```python
from build123d import *

# Parameters (mm, degrees)
SKETCH5_R           = 11
BOSS_EXTRUDE3_DEPTH = 3.84
SKETCH6_R           = 1.5
CUT_EXTRUDE16_DEPTH = 3.84
SKETCH6_8_R         = 2.9
SKETCH6_8_R_2       = 1.5
CUT_EXTRUDE17_DEPTH = 1
SKETCH7_R           = 0.75
CUT_EXTRUDE18_DEPTH = 2
SKETCH8_R           = 1.05
CUT_EXTRUDE20_DEPTH = 3
SKETCH8_4_R         = 1.25
SKETCH8_4_R_2       = 1.05
CUT_EXTRUDE21_DEPTH = 0.5
SKETCH15_W          = 0.299586516
SKETCH15_H          = 0.370347028
SKETCH15_W_2        = 0.300671414
CUT_EXTRUDE22_DEPTH = 3.84
SKETCH16_W          = 0.5
SKETCH16_H          = 0.298358963
CUT_EXTRUDE23_DEPTH = 3.84
SKETCH17_W          = 0.5
SKETCH17_H          = 1.60013733
CUT_EXTRUDE24_DEPTH = 0.25


with BuildPart() as part:
    # Sketch5 → Boss-Extrude3 (new body)
    with BuildSketch(Plane.XY):
        Circle(SKETCH5_R)
    extrude(amount=-BOSS_EXTRUDE3_DEPTH)

    # Sketch6 → Cut-Extrude16 (cut)
    with BuildSketch(Plane.XY):
        Circle(SKETCH6_R)
    extrude(amount=-CUT_EXTRUDE16_DEPTH, mode=Mode.SUBTRACT)

    # Sketch6<8> → Cut-Extrude17 (cut)
    with BuildSketch(Plane.XY):
        Circle(SKETCH6_8_R)
        Circle(SKETCH6_8_R_2, mode=Mode.SUBTRACT)
    extrude(amount=-CUT_EXTRUDE17_DEPTH, mode=Mode.SUBTRACT)

    # Sketch7 → Cut-Extrude18 (cut)
    with BuildSketch(Plane.XY):
        with Locations((-4.763139721, 2.75)):
            Circle(SKETCH7_R)
        with Locations((4.763139721, 2.75)):
            Circle(SKETCH7_R)
        with Locations((0, -5.5)):
            Circle(SKETCH7_R)
    extrude(amount=-CUT_EXTRUDE18_DEPTH, mode=Mode.SUBTRACT)

    # Sketch8 → Cut-Extrude20 (cut)
    with BuildSketch(Plane.XY):
        with Locations((-8, 0)):
            Circle(SKETCH8_R)
        with Locations((0, -8)):
            Circle(SKETCH8_R)
        with Locations((8, 0)):
            Circle(SKETCH8_R)
        with Locations((0, 8)):
            Circle(SKETCH8_R)
    extrude(amount=-CUT_EXTRUDE20_DEPTH, mode=Mode.SUBTRACT)

    # Sketch8<4> → Cut-Extrude21 (cut)
    # profile 1 of 4: a face of its own
    with BuildSketch(Plane.XY):
        with Locations((-8, 0)):
            Circle(SKETCH8_4_R)
        with Locations((-8, 0)):
            Circle(SKETCH8_4_R_2, mode=Mode.SUBTRACT)
    # profile 2 of 4: a face of its own
    with BuildSketch(Plane.XY):
        with Locations((0, -8)):
            Circle(SKETCH8_4_R)
        with Locations((0, -8)):
            Circle(SKETCH8_4_R_2, mode=Mode.SUBTRACT)
    # profile 3 of 4: a face of its own
    with BuildSketch(Plane.XY):
        with Locations((8, 0)):
            Circle(SKETCH8_4_R)
        with Locations((8, 0)):
            Circle(SKETCH8_4_R_2, mode=Mode.SUBTRACT)
    # profile 4 of 4: a face of its own
    with BuildSketch(Plane.XY):
        with Locations((0, 8)):
            Circle(SKETCH8_4_R)
        with Locations((0, 8)):
            Circle(SKETCH8_4_R_2, mode=Mode.SUBTRACT)
    extrude(amount=-CUT_EXTRUDE21_DEPTH, mode=Mode.SUBTRACT)

    # Sketch15 → Cut-Extrude22 (cut)
    with BuildSketch(Plane.XY):
        with Locations((-0.997080085, -10.814826486)):
            Rectangle(SKETCH15_W, SKETCH15_H)
        with Locations((1.003807665, -10.814826486)):
            Rectangle(SKETCH15_W_2, SKETCH15_H)
    extrude(amount=-CUT_EXTRUDE22_DEPTH, mode=Mode.SUBTRACT)

    # Sketch16 → Cut-Extrude23 (cut)
    with BuildSketch(Plane.XY):
        with Locations((0, 10.850819912)):
            Rectangle(SKETCH16_W, SKETCH16_H)
    extrude(amount=-CUT_EXTRUDE23_DEPTH, mode=Mode.SUBTRACT)

    # Sketch17 → Cut-Extrude24 (cut)
    with BuildSketch(Plane.XY):
        with Locations((0, 9.901571765)):
            Rectangle(SKETCH17_W, SKETCH17_H)
    extrude(amount=-CUT_EXTRUDE24_DEPTH, mode=Mode.SUBTRACT)


solid = part.part
```
Geometry: final body of the model. Coordinates: model frame, mm. A direction names the side the tool comes from. Give positions to 0.01 mm unless a question says otherwise; leave off trailing zeros. Write each loop counter-clockwise with the first axis right and the second up, starting at its lowest first coordinate (ties: lowest second). Pieces come first, ordered by that corner, then holes.
1. Section query A-A, the plane z = -1.5. Count the separate pieces of the cut face and the enclosed holes in it, then the cut area to 3 significant figures.
2. Section query C-C, the plane x = 8. Return loops of the section in (y, z), then the cut area to 3 significant figures.
3. Section query B-B, the plane y = 0. Return loops of the section in (x, z).
4. Reachability of faces 1 (the cylindrical face through (0.56, 8.89, -1.73)), 2 (the cylindrical face through (-1.5, 0.07, -2.4)) from +Z, -Z, +X, -X, +Y, -Y: full face, straight path, thin tool, end or side. Return the list, or none.
5. Line query: probe 1 along Y at (x, z) = (0, -1.5); probe 2 along Y at (x, z) = (-6.25, -2.95); probe 3 along Y at (x, z) = (0.5, -2.9). Output: solid intervals per line, ascending.
6. Pin query (flat end, axial travel): P1, Ø1, axis at x = -8, y = 0, coming from the +Z side; P2, Ø2, axis at x = -4.5, z = -2.5, coming from the +Y side; P3, Ø0.6, axis at x = 0, z = -2.5, coming from the +Y side; P4, Ø1, axis at y = 3.5, z = -2.5, coming from the -X side. Return the tip coordinate at first contact, or that it passes through.
7. Draft query along X for faces 3 (the flat face through (1.2, -1.2, -1)), 4 (the flat face through (2.3, -2.3, 0)), 5 (the cylindrical face through (-10.98, 0.68, -1.89)), 6 (the flat face through (-8, 0, -3)). Return one class per face: released by +X, released by -X, zero draft, split by the parting line, or undercut.
Computed:
1. separate pieces: 1
1. enclosed holes: 8
1. area: 354 mm2
2. outline: (-7.55, -3.84) - (7.55, -3.84) - (7.55, 0) - (1.25, 0) - (1.25, -0.5) - (1.05, -0.5) - (1.05, -3) - (-1.05, -3) - (-1.05, -0.5) - (-1.25, -0.5) - (-1.25, 0) - (-7.55, 0) - close
2. area: 51.5 mm2
3. outline: (-11, -3.84) - (-1.5, -3.84) - (-1.5, -1) - (-2.9, -1) - (-2.9, 0) - (-6.75, 0) - (-6.75, -0.5) - (-6.95, -0.5) - (-6.95, -3) - (-9.05, -3) - (-9.05, -0.5) - (-9.25, -0.5) - (-9.25, 0) - (-11, 0) - close; (1.5, -3.84) - (11, -3.84) - (11, 0) - (9.25, 0) - (9.25, -0.5) - (9.05, -0.5) - (9.05, -3) - (6.95, -3) - (6.95, -0.5) - (6.75, -0.5) - (6.75, 0) - (2.9, 0) - (2.9, -1) - (1.5, -1) - close
4. face 1: +Z
4. face 2: +Z, -Z
5. probe 1: y = -11 to -9.05, -6.95 to -6.25, -4.75 to -1.5, 1.5 to 6.95, 9.05 to 10.7
5. probe 2: y = -9.05 to 9.05
5. probe 3: y = -10.99 to -8.92, -7.08 to -1.41, 1.41 to 7.08, 8.92 to 10.99
6. P1: stops at z = -3
6. P2: stops at y = 10.43
6. P3: stops at y = 11
6. P4: stops at x = -10.58
7. face 3: undercut
7. face 4: zero draft
7. face 5: released by -X
7. face 6: undercut
